Read the model definition and answer for the solid it produces. Units are mm, in the model's axes. Face numbers are marked on the shaded views. Give positions to 0.01 mm unless a question says otherwise; leave off trailing zeros. Order: outer loops, then holes, each group sorted by start corner. A loop starts at its lowest first (then second) coordinate and runs counter-clockwise, first axis right, second up. Notation, with made-up numbers: M 61,-40 L 95,-40 A30 cw 95,-9 Z; hole C -22,-17.5 d11. An arc over 180 degrees is marked long. One line per item, written item: value.
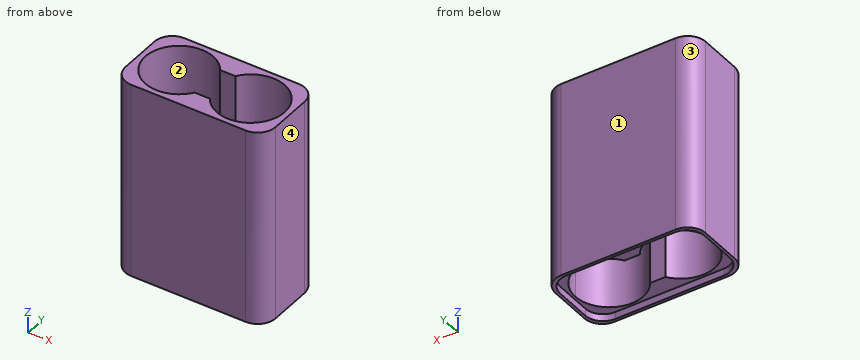
from build123d import *

# Parameters (mm, degrees)
F0_W     = 42
F0_H     = 22
F1_DEPTH = 55
F2_W     = 40.4
F2_H     = 20.4
F3_DEPTH = 2
F4_R     = 5


with BuildPart() as f1:
    # F0 (on Top) → F1 (new body)
    with BuildSketch(Plane.XY):
        Rectangle(F0_W, F0_H)
        with BuildLine():
            ThreePointArc((-2.120368, -5.306732), (-19.5, 0), (-2.120368, 5.306732))
            Line((-2.120368, 5.306732), (2.120368, 5.306732))
            ThreePointArc((2.120368, 5.306732), (12.774302, 9.085882), (19.5, 0))
            ThreePointArc((19.5, 0), (12.774302, -9.085882), (2.120368, -5.306732))
            Line((2.120368, -5.306732), (-2.120368, -5.306732))
        make_face(mode=Mode.SUBTRACT)
    extrude(amount=F1_DEPTH)

    # F2 (on face) → F3 (cut)
    with BuildSketch(Plane(origin=(0, 0, 0), x_dir=(1, 0, 0), z_dir=(0, 0, -1))):
        Rectangle(F2_W, F2_H)
    extrude(amount=-F3_DEPTH, mode=Mode.SUBTRACT)

    # F4
    f4_edges = [f1.edges().sort_by_distance(p)[0] for p in [
        (-20.2, -10.2, 1),
        (20.2, -10.2, 1),
        (20.2, 10.2, 1),
        (-20.2, 10.2, 1),
        (21, -11, 27.5),
        (-21, -11, 27.5),
        (21, 11, 27.5),
        (-21, 11, 27.5),
    ]]
    fillet(f4_edges, radius=F4_R)


solid = f1.part
1) Consider probe 1 along X at (y, z) = (7, 20); probe 2 along Y at (x, z) = (-10, 35); probe 3 along X at (y, z) = (-5.5, 31.5). Determine where each line is inside the solid, lowest interval first.
Reported:
probe 1: x = -20.9 to -16.42, -3.58 to 3.58, 16.42 to 20.9
probe 2: y = -11 to -9.5, 9.5 to 11
probe 3: x = -21 to -17.75, -2.25 to 2.25, 17.75 to 21
2) Find section C-C, the plane z = 24. Write down the section's boundary in (x, y), plus the area to 3 significant figures.
Reported:
outline: M -21,-6 A5 ccw -16,-11 L 16,-11 A5 ccw 21,-6 L 21,6 A5 ccw 16,11 L -16,11 A5 ccw -21,6 Z; hole M -2.12,-5.31 L 2.12,-5.31 A9.5 ccw long 2.12,5.31 L -2.12,5.31 A9.5 ccw long Z
area: 314 mm^2
3) Determine the mould class of the marked faces 1, 2, 3 and 4 for opening direction X: +X half, -X half, draft (parallel to the pull), parting line (faces both ways), or undercut.
Reported:
face 1: draft
face 2: undercut
face 3: -X half
face 4: +X half
4) Find section B-B, the plane y = 4. Write down the section's boundary in (x, z), plus the area to 3 significant figures.
Reported:
outline: M -21,0 L -20.2,0 L -20.2,2 L -18.62,2 L -18.62,55 L -21,55 Z; M 18.62,2 L 20.2,2 L 20.2,0 L 21,0 L 21,55 L 18.62,55 Z
area: 256 mm^2
5) Find section A-A, the plane x = -1.5. Write down the section's boundary in (y, z), plus the area to 3 significant figures.
Reported:
outline: M -11,0 L -10.2,0 L -10.2,2 L -5.31,2 L -5.31,55 L -11,55 Z; M 5.31,2 L 10.2,2 L 10.2,0 L 11,0 L 11,55 L 5.31,55 Z
area: 607 mm^2
